Here's how the part is built. I have some questions about the finished solid (model axes, mm). A direction names the side the tool comes from. Round coordinates to 2 decimals unless told otherwise and drop trailing zeros. Loops run counter-clockwise (first coordinate to the right, second up) from the corner with the lowest first, then second, coordinate; pieces in that order, holes last. Notation, with made-up numbers: M -0.75,46.5 L 27.25,46.5 A31 cw 27.25,83.5 Z; hole C 60.25,4 d4. An arc over 180 degrees is marked long. Answer as CSV lines item,"result".
```python
from build123d import *

# Parameters (mm, degrees)
F1_DEPTH = 5
F2_R     = 1.487565
F3_DEPTH = 25


with BuildPart() as f1:
    # F0 (on Top) → F1 (new body)
    with BuildSketch(Plane.XY):
        with BuildLine():
            ThreePointArc((-14.500521, 15.723383), (-15.72616, 14.852099), (-16.19577, 13.423536))
            Line((-16.19577, 13.423536), (-16.19577, -14.155729))
            ThreePointArc((-16.19577, -14.155729), (-15.580113, -15.265987), (-14.515248, -15.957195))
            Line((-14.515248, -15.957195), (13.538033, -15.957195))
            ThreePointArc((13.538033, -15.957195), (14.664759, -15.140462), (15.249531, -13.877685))
            Line((15.249531, -13.877685), (15.249531, 13.492324))
            ThreePointArc((15.249531, 13.492324), (14.531055, 14.889514), (13.19951, 15.723383))
            Line((13.19951, 15.723383), (-14.500521, 15.723383))
        make_face()
        Polygon((-9.889765, 0), (-12.746189, 0), (-12.965441, 0), (-12.965441, -0.315834), (-12.965441, -2.466221), (-9.700684, -2.466221), (-9.700684, -2.596811), (-9.889765, -2.997288), (-9.987982, -3.110466), (-10.214339, -3.180114), (-13.522626, -3.180114), (-13.818631, -3.110466), (-13.968735, -2.727133), (-13.968735, 0.355315), (-13.660931, 0.671027), (-13.192589, 0.790616), (-10.528548, 0.790616), (-9.889765, 0.355315), align=None, mode=Mode.SUBTRACT)
        Polygon((-8.720032, 0.355315), (-8.110611, 0.790616), (-5.376921, 0.790616), (-4.279962, 0), (-7.919079, 0), (-7.919079, -0.77241), (-4.941619, -0.77241), (-4.279962, -1.329595), (-4.279962, -2.727133), (-4.610791, -3.175272), (-8.128023, -3.175272), (-8.789681, -2.727133), (-8.789681, -2.466221), (-5.150564, -2.466221), (-5.150564, -1.764896), (-5.324685, -1.608188), (-8.302143, -1.608188), (-8.720032, -1.207711), (-8.720032, 0), align=None, mode=Mode.SUBTRACT)
        Polygon((4.463568, -1.329595), (4.463568, -1.069831), (7.363056, -0.965359), (7.363056, -2.727133), (7.075374, -3.175272), (3.186837, -3.175272), (2.913897, -2.727133), (2.913897, 0.343786), (3.418846, 0.790616), (6.692736, 0.790616), (7.388791, 0.343786), (7.388791, 0), (3.767087, 0), (3.767087, -2.532442), (6.448541, -2.532442), (6.448541, -1.634477), (4.9385, -1.634477), align=None, mode=Mode.SUBTRACT)
        Polygon((8.903638, 0.790616), (12.002981, 0.790616), (12.551844, 0.343786), (12.551844, -2.727133), (12.264162, -3.175272), (8.693178, -3.175272), (8.207156, -2.863271), (8.207156, 0), align=None, mode=Mode.SUBTRACT)
        with BuildLine():
            Line((0.510285, 4.991175), (0.510285, 4.822795))
            Line((0.510285, 4.822795), (1.027232, 4.781501))
            Line((1.027232, 4.781501), (1.027232, 4.970423))
            Line((1.027232, 4.970423), (1.443637, 5.0924))
            Line((1.443637, 5.0924), (1.547077, 4.739275))
            Line((1.547077, 4.739275), (4.141693, 4.739275))
            Line((4.141693, 4.739275), (4.244784, 4.57001))
            Line((4.244784, 4.57001), (5.379676, 4.57001))
            Line((5.379676, 4.57001), (5.379676, 4.269563))
            Line((5.379676, 4.269563), (4.282718, 4.269563))
            Line((4.282718, 4.269563), (2.941991, 4.269563))
            Line((2.941991, 4.269563), (2.744667, 3.93836))
            Line((2.744667, 3.93836), (2.345195, 3.69506))
            Line((2.345195, 3.69506), (2.562487, 3.338289))
            Line((2.562487, 3.338289), (2.658973, 3.179869))
            Line((2.658973, 3.179869), (2.493863, 3.079309))
            Line((2.493863, 3.079309), (2.332569, 2.981072))
            Line((2.332569, 2.981072), (1.877723, 2.421154))
            Line((1.877723, 2.421154), (1.6535, 2.284591))
            Line((1.6535, 2.284591), (1.443637, 2.284591))
            Line((1.443637, 2.284591), (0.811452, 2.69042))
            Line((0.811452, 2.69042), (0.625802, 2.57735))
            Line((0.625802, 2.57735), (0.782898, 2.319415))
            Line((0.782898, 2.319415), (0.782898, 0.790616))
            Line((0.782898, 0.790616), (0.347854, 0.790616))
            Line((0.347854, 0.790616), (0.347854, 0.430846))
            Line((0.347854, 0.430846), (1.443637, -1.634477))
            Line((1.443637, -1.634477), (1.23433, -4.306218))
            Line((1.23433, -4.306218), (2.120807, -5.039395))
            Line((2.120807, -5.039395), (0.369284, -5.039395))
            Line((0.369284, -5.039395), (0.244222, -4.834056))
            Line((0.244222, -4.834056), (0.544849, -4.650959))
            Line((0.544849, -4.650959), (0.544849, -3.641361))
            Line((0.544849, -3.641361), (0.273981, -3.444366))
            Line((0.273981, -3.444366), (0.273981, -2.727133))
            Line((0.273981, -2.727133), (0.458664, -1.99153))
            Line((0.458664, -1.99153), (0, -1.585228))
            Line((0, -1.585228), (-1.031109, -0.77241))
            Line((-1.031109, -0.77241), (-1.445959, -1.548292))
            Line((-1.445959, -1.548292), (-2.003771, -2.385519))
            Line((-2.003771, -2.385519), (-1.858417, -2.914943))
            Line((-1.858417, -2.914943), (-2.845868, -4.380091))
            Line((-2.845868, -4.380091), (-2.845868, -4.834056))
            Line((-2.845868, -4.834056), (-2.601957, -5.234533))
            Line((-2.601957, -5.234533), (-3.437877, -5.234533))
            Line((-3.437877, -5.234533), (-3.437877, -4.86888))
            Line((-3.437877, -4.86888), (-3.437877, -4.468403))
            Line((-3.437877, -4.468403), (-3.209849, -3.841491))
            Line((-3.209849, -3.841491), (-3.296034, -3.373629))
            Line((-3.296034, -3.373629), (-3.135976, -3.065825))
            Line((-3.135976, -3.065825), (-3.025166, -2.881142))
            Line((-3.025166, -2.881142), (-3.025166, -2.400967))
            Line((-3.025166, -2.400967), (-2.601957, -1.994665))
            Line((-2.601957, -1.994665), (-2.601957, -0.874258))
            Line((-2.601957, -0.874258), (-2.458807, -0.77241))
            Line((-2.458807, -0.77241), (-2.458807, -0.418708))
            Line((-2.458807, -0.418708), (-2.601957, -0.32021))
            Line((-2.601957, -0.32021), (-2.601957, 0.343786))
            Line((-2.601957, 0.343786), (-2.305952, 0.430846))
            Line((-2.305952, 0.430846), (-2.305952, 1.710631))
            Line((-2.305952, 1.710631), (-2.500045, 1.710631))
            Line((-2.500045, 1.710631), (-2.500045, 2.899405))
            Line((-2.500045, 2.899405), (-1.858417, 2.899405))
            Line((-1.858417, 2.899405), (-1.858417, 3.317294))
            Line((-1.858417, 3.317294), (-2.007655, 3.385334))
            Line((-2.007655, 3.385334), (-2.099568, 3.491414))
            Line((-2.099568, 3.491414), (-1.858417, 3.700359))
            Line((-1.858417, 3.700359), (-1.858417, 4.424379))
            Line((-1.858417, 4.424379), (-1.445959, 4.892242))
            Line((-1.445959, 4.892242), (-0.836507, 4.892242))
            ThreePointArc((-0.836507, 4.892242), (-0.739639, 4.970476), (-0.714366, 5.0924))
            ThreePointArc((-0.714366, 5.0924), (-0.749437, 5.530727), (-0.533184, 5.913604))
            ThreePointArc((-0.533184, 5.913604), (-0.011449, 6.109638), (0.510285, 5.913604))
            Line((0.510285, 5.913604), (0.627419, 5.811112))
            Line((0.627419, 5.811112), (0.773836, 5.693978))
            Line((0.773836, 5.693978), (0.773836, 5.525598))
            Line((0.773836, 5.525598), (0.773836, 5.357218))
            Line((0.773836, 5.357218), (0.773836, 5.210801))
            Line((0.773836, 5.210801), (0.627419, 5.079025))
            Line((0.627419, 5.079025), (0.510285, 4.991175))
        make_face(mode=Mode.SUBTRACT)
    extrude(amount=F1_DEPTH)

    # F2 (on face) → F3 (cut)
    with BuildSketch(Plane.XY.offset(5)):
        with Locations((12.347989, 12.883592)):
            Circle(F2_R)
    extrude(amount=-F3_DEPTH, mode=Mode.SUBTRACT)


solid = f1.part
```
1. I want a section at B-B, the plane z = 4.25. Count the separate pieces of the cut face and the enclosed holes in it, and give its area (3 significant figures).
Evaluation:
separate pieces,"1"
enclosed holes,"6"
area,"905 mm²"
2. We'd pull the mould along Y, two halves only. Please class faces 1 (the flat face through (15.25, 0, 2)), 2 (the cylindrical face through (14.55, 14.87, 2.46)), 3 (the cylindrical face through (-0.75, 5.52, 2.46)): pulls with the +Y half, pulls with the -Y half, needs draft (parallel to the pull), parting line crosses it, or undercut.
Evaluation:
face 1,"needs draft"
face 2,"pulls with the +Y half"
face 3,"undercut"
3. Which directions (+Z, -Z, +X, -X, +Y, -Y) give clear straight access to the entire face, cutting with the end or side of a thin tool? Please do faces 4 (the cylindrical face through (-15.592, -15.253, 2.465)), 5 (the flat face through (6.449, -2, 2)).
Evaluation:
face 4,"+Z, -Z, -X, -Y"
face 5,"+Z, -Z"
4. If I drill on line 1 (Y direction, x = -8, z = 3.5); line 2 (Y direction, x = -6.5, z = 1.8); line 3 (Y direction, x = 10, z = 4.45), over which ranges is the centre line in solid material (lowest first)? Write a range as [from, to].
Evaluation:
line 1,"y = [-15.96, -3.18], [-2.47, -1.61], [0.79, 15.72]"
line 2,"y = [-15.96, -3.18], [-2.47, -1.61], [-0.77, 0], [0.79, 15.72]"
line 3,"y = [-15.96, -3.18], [0.79, 15.72]"
5. I want a section at A-A, the plane y = 12. Please give me the cut outline in (x, z), and give its area (3 significant figures).
Evaluation:
outline,"M -16.2,0 L 11.15,0 L 11.15,5 L -16.2,5 Z; M 13.54,0 L 15.25,0 L 15.25,5 L 13.54,5 Z"
area,"145 mm²"
